```python
from build123d import *

# Parameters (mm, degrees)
F0_W      = 78.04359
F0_H      = 105.09279
F0_R      = 16.850319
F1_DEPTH  = 2.54
F2_W      = 78.04359
F2_H      = 21.505939
F3_DEPTH  = 2.54
F4_W      = 78.04359
F4_H      = 21.21968
F5_DEPTH  = 2.54
F7_DEPTH  = 2.54
F8_W      = 100.01279
F8_H      = 21.21968
F9_DEPTH  = 2.54
F10_W     = 17.748192
F10_H     = 8.874096
F11_DEPTH = 7.62


with BuildPart() as f1:
    # F0 (on Top) → F1 (new body)
    with BuildSketch(Plane.XY):
        with Locations((19.510894, 11.085736)):
            Rectangle(F0_W, F0_H)
        with Locations((40.35208, 39.243508)):
            Circle(F0_R, mode=Mode.SUBTRACT)
    extrude(amount=F1_DEPTH)

    # F2 (on face) → F3 (join)
    with BuildSketch(Plane(origin=(0, 63.632131, 0), x_dir=(-1, 0, 0), z_dir=(0, 1, 0))):
        with Locations((-19.510894, 13.292969)):
            Rectangle(F2_W, F2_H)
    extrude(amount=-F3_DEPTH)

    # F4 (on face) → F5 (join)
    with BuildSketch(Plane.XZ.offset(41.460659)):
        with Locations((19.510894, 13.14984)):
            Rectangle(F4_W, F4_H)
    extrude(amount=-F5_DEPTH)

    # F6 (on face) → F7 (join)
    with BuildSketch(Plane(origin=(-19.510901, 0, 0), x_dir=(0, -1, 0), z_dir=(-1, 0, 0))):
        Polygon((38.920659, 24.045939), (-61.092131, 24.045939), (-61.092131, 2.54), (38.920659, 2.54), (38.920659, 23.75968), align=None)
    extrude(amount=-F7_DEPTH)

    # F8 (on face) → F9 (join)
    with BuildSketch(Plane.YZ.offset(58.532689)):
        with Locations((11.085736, 13.14984)):
            Rectangle(F8_W, F8_H)
    extrude(amount=-F9_DEPTH)

    # F10 (on face) → F11 (join)
    with BuildSketch(Plane(origin=(-19.510901, 0, 0), x_dir=(0, -1, 0), z_dir=(-1, 0, 0))):
        with Locations((-29.05551, 12.738623)):
            Rectangle(F10_W, F10_H)
    extrude(amount=F11_DEPTH)


solid = f1.part
```
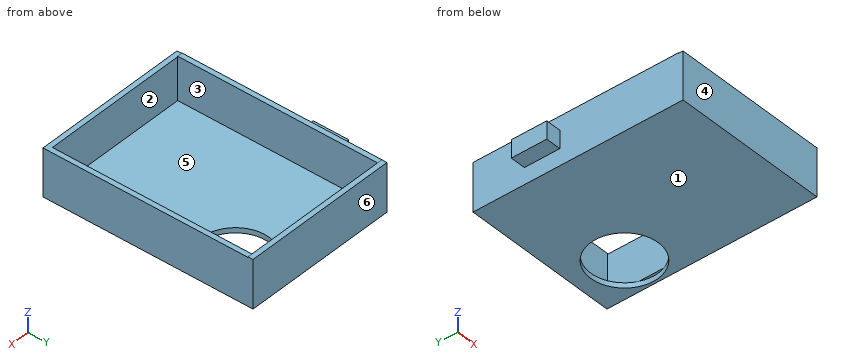
Geometry check sheet. Reference: the model listing, model coordinates, mm. Face numbers are marked on the shaded views. A direction names the side the tool comes from. Give positions to 0.01 mm unless a question says otherwise; leave off trailing zeros. Order: outer loops, then holes, each group sorted by start corner. A loop starts at its lowest first (then second) coordinate and runs counter-clockwise, first axis right, second up. Notation, with made-up numbers: (-31.75, 29) - (6.25, 29) arc R19 cw to (6.25, 65) - close; hole circle Ø2 at (16.25, -38). An arc over 180 degrees is marked (long way). Write item = value, one per line. Start each with the question number.
1) Section check B-B (x = 4). Enter the section's corners in (y, z), then the cut area to 3 significant figures.
2) Section check A-A (z = 19). Enter the section's corners in (x, y).
3) Section check D-D (x = 36.5). Enter the section's corners in (y, z).
4) Access from +Z, -Z, +X, -X, +Y, -Y to the whole of each face (thin tool, end or side, straight path). Record for the marked faces 1 and 2.
5) Section check C-C (y = 34.5). Enter the section's corners in (x, z), then the cut area to 3 significant figures.
6) Gauge pin test, flat ends, axial feed: pin 1 Ø8.5 at (x, y) = (-23.5, 25) entering from -Z; pin 2 Ø6 at (x, y) = (44.5, 1.5) entering from +Z; pin 3 Ø6.5 at (y, z) = (3, 13.5) entering from -X. Record the tip position at first contact, or that the pin passes through.
7) Draft check along Y on the marked faces 3, 4, 5 and 6. Enter one of: released by +Y, released by -Y, zero draft, split by the parting line, or undercut.
8) Scan lines: L1, parallel to X at y = 23, z = 18; L2, parallel to Y at x = 16.5, z = 13; L3, parallel to Z at x = -5.5, y = 54.5. Record each from-to range of solid material in increasing order.
Geometry check:
q1.outline = (-41.46, 0) - (63.63, 0) - (63.63, 24.05) - (61.09, 24.05) - (61.09, 2.54) - (-38.92, 2.54) - (-38.92, 23.76) - (-41.46, 23.76) - close
q1.area = 375 mm2
q2.outline = (-19.51, -41.46) - (58.53, -41.46) - (58.53, 63.63) - (-19.51, 63.63) - close; hole (-16.97, -38.92) - (55.99, -38.92) - (55.99, 61.09) - (-16.97, 61.09) - close
q3.outline = (-41.46, 0) - (22.84, 0) - (22.84, 2.54) - (-38.92, 2.54) - (-38.92, 23.76) - (-41.46, 23.76) - close; (55.65, 0) - (63.63, 0) - (63.63, 24.05) - (61.09, 24.05) - (61.09, 2.54) - (55.65, 2.54) - close
q4.face_1 = -Z, +X, -X, +Y, -Y
q4.face_2 = +Z
q5.outline = (-27.13, 8.3) - (-19.51, 8.3) - (-19.51, 0) - (24.18, 0) - (24.18, 2.54) - (-16.97, 2.54) - (-16.97, 24.05) - (-19.51, 24.05) - (-19.51, 17.18) - (-27.13, 17.18) - close; (55.99, 2.54) - (56.52, 2.54) - (56.52, 0) - (58.53, 0) - (58.53, 23.76) - (55.99, 23.76) - close
q5.area = 292 mm2
q6.pin_1 = 0
q6.pin_2 = 2.54
q6.pin_3 = -19.51
q7.face_3 = undercut
q7.face_4 = released by -Y
q7.face_5 = undercut
q7.face_6 = released by +Y
q8.L1 = -19.51 to -16.97, 55.99 to 58.53
q8.L2 = -41.46 to -38.92, 61.09 to 63.63
q8.L3 = 0 to 2.54
